The listing builds one solid part. Answer for the finished solid, in the listing's coordinates (mm). A direction names the side the tool comes from. Round coordinates to 2 decimals unless told otherwise and drop trailing zeros. Write each loop counter-clockwise with the first axis right and the second up, starting at its lowest first coordinate (ties: lowest second). Pieces come first, ordered by that corner, then holes. Notation, with made-up numbers: (-28, 58) - (7, 58) arc R8 cw to (7, 63) - close; hole circle Ø9 at (1.25, 86.5). An arc over 180 degrees is marked (long way). Answer in a Markdown table with one row per item.
from build123d import *

# Parameters (mm, degrees)
SKETCH1_W           = 101.6
SKETCH1_H           = 101.6
BOSS_EXTRUDE1_DEPTH = 3.175
SKETCH2_W           = 101.6
SKETCH2_H           = 101.6
SKETCH2_W_2         = 88.9
SKETCH2_H_2         = 88.9
BOSS_EXTRUDE2_DEPTH = 6.35
SKETCH3_R           = 0.99949
CUT_EXTRUDE1_DEPTH  = 6.35
CIRPATTERN1_COUNT   = 4
SKETCH4_W           = 101.6
SKETCH4_H           = 101.6
SKETCH4_W_2         = 95.25
SKETCH4_H_2         = 95.25
CUT_EXTRUDE2_DEPTH  = 9.525
SKETCH5_R           = 1.905
SKETCH5_R_2         = 0.99949
BOSS_EXTRUDE3_DEPTH = 3.175
SKETCH6_R           = 0.99949
CUT_EXTRUDE3_DEPTH  = 7.35
CHAMFER1_SIZE       = 1.27
CHAMFER2_SIZE       = 1.27


with BuildPart() as part:
    # Sketch1 → Boss-Extrude1 (new body)
    with BuildSketch(Plane(origin=(0, 0, 0), x_dir=(1, 0, 0), z_dir=(0, 1, 0))):
        Rectangle(SKETCH1_W, SKETCH1_H)
    extrude(amount=BOSS_EXTRUDE1_DEPTH)

    # Sketch2 → Boss-Extrude2 (add)
    with BuildSketch(Plane(origin=(0, 3.175, 0), x_dir=(1, 0, 0), z_dir=(0, 1, 0))):
        Rectangle(SKETCH2_W, SKETCH2_H)
        Rectangle(SKETCH2_W_2, SKETCH2_H_2, mode=Mode.SUBTRACT)
    extrude(amount=BOSS_EXTRUDE2_DEPTH)

    # Sketch3 → Cut-Extrude1 (cut)
    with BuildSketch(Plane.XY.offset(50.8)):
        with Locations((-38.1, 6.35)):
            Circle(SKETCH3_R)
        with Locations((38.1, 6.35)):
            Circle(SKETCH3_R)
    cut_extrude1 = extrude(amount=-CUT_EXTRUDE1_DEPTH, mode=Mode.SUBTRACT)

    # CirPattern1: Cut-Extrude1 ×4 about axis
    cirpattern1_axis = Axis((0, 10.00125, 0), (0, -1, 0))
    for i in range(1, CIRPATTERN1_COUNT):
        add(cut_extrude1.rotate(cirpattern1_axis, i * 360 / CIRPATTERN1_COUNT), mode=Mode.SUBTRACT)

    # Sketch4 → Cut-Extrude2 (cut)
    with BuildSketch(Plane(origin=(0, 0, 0), x_dir=(1, 0, 0), z_dir=(0, 1, 0))):
        Rectangle(SKETCH4_W, SKETCH4_H)
        Rectangle(SKETCH4_W_2, SKETCH4_H_2, mode=Mode.SUBTRACT)
    extrude(amount=CUT_EXTRUDE2_DEPTH, mode=Mode.SUBTRACT)

    # Sketch5 → Boss-Extrude3 (add)
    with BuildSketch(Plane(origin=(0, 3.175, 0), x_dir=(1, 0, 0), z_dir=(0, 1, 0))):
        with Locations((-35.052, -35.052)):
            Circle(SKETCH5_R)
        with Locations((-35.052, -35.052)):
            Circle(SKETCH5_R_2, mode=Mode.SUBTRACT)
        with Locations((35.052, -35.052)):
            Circle(SKETCH5_R)
        with Locations((35.052, -35.052)):
            Circle(SKETCH5_R_2, mode=Mode.SUBTRACT)
        with Locations((35.052, 35.052)):
            Circle(SKETCH5_R)
        with Locations((35.052, 35.052)):
            Circle(SKETCH5_R_2, mode=Mode.SUBTRACT)
        with Locations((-35.052, 35.052)):
            Circle(SKETCH5_R)
        with Locations((-35.052, 35.052)):
            Circle(SKETCH5_R_2, mode=Mode.SUBTRACT)
    extrude(amount=BOSS_EXTRUDE3_DEPTH)

    # Sketch6 → Cut-Extrude3 (cut, through all)
    with BuildSketch(Plane(origin=(0, 6.35, 0), x_dir=(1, 0, 0), z_dir=(0, 1, 0))):
        with Locations((-35.052, 35.052)):
            Circle(SKETCH6_R)
        with Locations((35.052, 35.052)):
            Circle(SKETCH6_R)
        with Locations((35.052, -35.052)):
            Circle(SKETCH6_R)
        with Locations((-35.052, -35.052)):
            Circle(SKETCH6_R)
    extrude(amount=-CUT_EXTRUDE3_DEPTH, mode=Mode.SUBTRACT)

    # Chamfer1
    chamfer1_edges = [part.edges().sort_by_distance(p)[0] for p in [
        (-36.05149, 0, 35.052),
        (34.05251, 0, 35.052),
        (34.05251, 0, -35.052),
        (-36.05149, 0, -35.052),
    ]]
    chamfer(chamfer1_edges, length=CHAMFER1_SIZE)

    # Chamfer2
    chamfer2_edges = [part.edges().sort_by_distance(p)[0] for p in [
        (-36.957, 3.175, 35.052),
        (33.147, 3.175, 35.052),
        (33.147, 3.175, -35.052),
        (-36.957, 3.175, -35.052),
    ]]
    chamfer(chamfer2_edges, length=CHAMFER2_SIZE)


solid = part.part
(1) Section A-A (x = -11) is taken. Give the vertices of the cut face in (y, z) (3 decimals).
Checked values:
| item | result |
|---|---|
| outline | (0, -47.625) - (9.525, -47.625) - (9.525, -44.45) - (3.175, -44.45) - (3.175, 44.45) - (9.525, 44.45) - (9.525, 47.625) - (0, 47.625) - close |
(2) Find the intervals of material crossed by line 1 (Y direction, x = 45, z = 38) (3 decimals); line 2 (Z direction, x = -12, y = 5.5) (3 decimals), in increasing order.
Checked values:
| item | result |
|---|---|
| line 1 | y = 0 to 5.356, 7.344 to 9.525 |
| line 2 | z = -47.625 to -44.45, 44.45 to 47.625 |
(3) Flat-ended cylindrical pins translate along their axes: pin 1 (1.2 mm diameter, centred on x = -38.1, y = 6.35, fed in from +Z); pin 2 (2.5 mm diameter, centred on y = 6.35, z = -38.1, fed in from +X) (3 decimals); pin 3 (1.1 mm diameter, centred on x = -34.5, z = -34.5, fed in from +Y). Find the tip coordinate at first contact, or state that the pin passes through.
Checked values:
| item | result |
|---|---|
| pin 1 | passes through |
| pin 2 | stops at x = 47.625 |
| pin 3 | stops at y = 6.35 |
(4) Section B-B (z = 3.5) is taken. Give the vertices of the cut face in (x, y) (3 decimals), and give its area (3 significant figures).
Checked values:
| item | result |
|---|---|
| outline | (-47.625, 0) - (47.625, 0) - (47.625, 9.525) - (44.45, 9.525) - (44.45, 3.175) - (-44.45, 3.175) - (-44.45, 9.525) - (-47.625, 9.525) - close |
| area | 343 mm2 |
(5) For faces 5 (the cylindrical face through (36.076, 5.384, -36.658)), 6 (the flat face through (-1, 5, 47.625)), determine the directions among +Z, -Z, +X, -X, +Y, -Y from which every point of the face is accessible in a straight line to the end or side of a thin tool.
Checked values:
| item | result |
|---|---|
| face 5 | +Y |
| face 6 | +Z, +X, -X, +Y, -Y |
(6) For a pull along X with two mould halves and no side action, classify faces 1 (the flat face through (-34, 6.35, -34)), 2 (the flat face through (47.625, 5, 1)), 3 (the flat face through (-1, 0, -1)), 4 (the flat face through (-47.625, 5, 1)) as pulls with the +X half, pulls with the -X half, needs draft (parallel to the pull), parting line crosses it, or undercut.
Checked values:
| item | result |
|---|---|
| face 1 | undercut |
| face 2 | pulls with the +X half |
| face 3 | needs draft |
| face 4 | pulls with the -X half |
